Part print with two shaded views. Sizes in mm from the minimum x, y, z corner. A direction names the side the tool comes from. Give positions to 0.01 mm unless a question says otherwise; leave off trailing zeros. Order: outer loops, then holes, each group sorted by start corner. A loop starts at its lowest first (then second) coordinate and runs counter-clockwise, first axis right, second up. Notation, with made-up numbers: (70, -15.5) -> (127, -15.5) arc R17 cw to (127, -2.5) -> close; hole circle Ø4 at (-17.75, 39.5). An arc over 180 degrees is marked (long way). Write item = value, one per line. Start each with the question number.
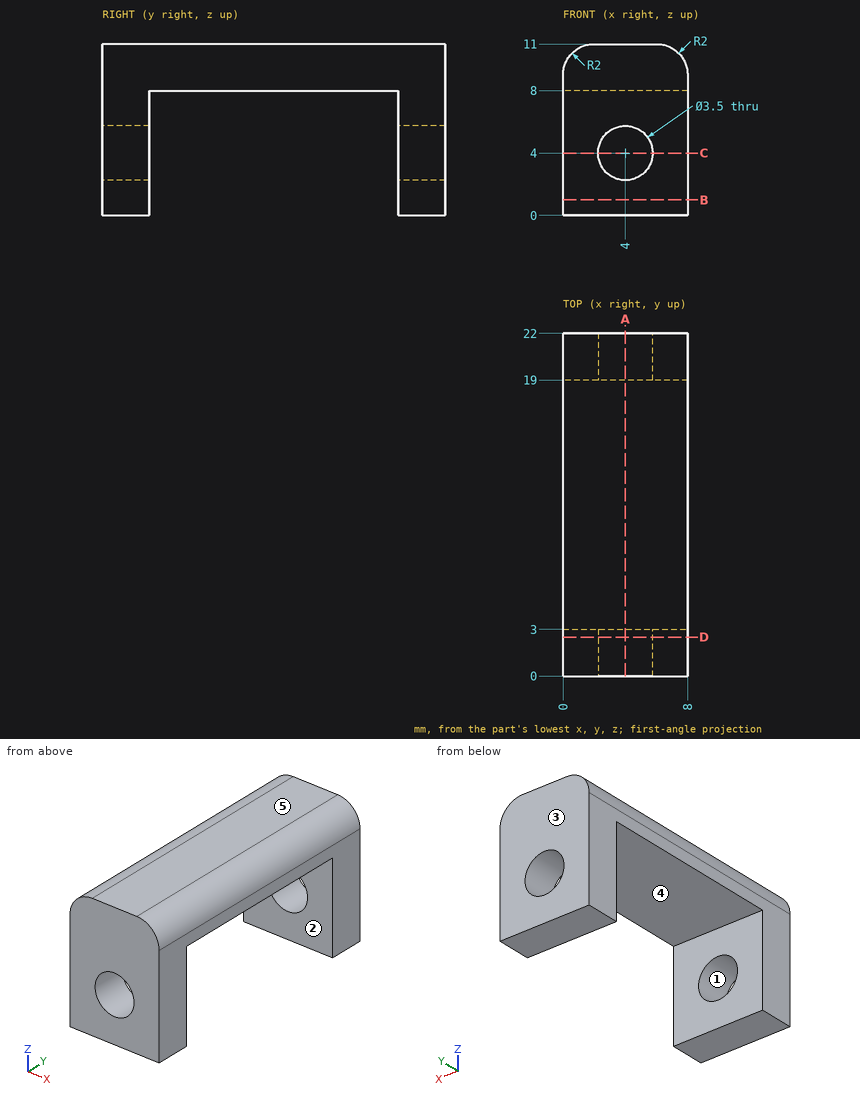
(1) Flat gauge pins, fed straight in: P1, Ø4, axis at x = 7, y = 15, coming from the +Z side; P2, Ø1, axis at x = 1, y = 9, coming from the -Z side. Where does each tip first touch, or does it go through?
(2) Cut at B-B, the plane z = 1. Give the cut face in (x, y).
(3) Cut at A-A, the plane x = 4. Give the cut face in (y, z).
(4) Cut at C-C, the plane z = 4. Give the cut face in (x, y), plus the area to 3 significant figures.
(5) 3-axis set-ups, long thin cutter, end or side, ignore diameter. For the marked faces 4 and 5: which of +Z, -Z, +X, -X, +Y, -Y reach the whole face in a straight line?
(6) Wall check: line 1 (Z direction, x = 4, y = 19.95); line 2 (Y direction, x = 1.75, z = 2.25); line 3 (X direction, y = 21.3, z = 4). Give the ranges that are in metal, low to high. Write a range as [from, to].
(7) Cut at D-D, the plane y = 2.5. Give the cut face in (x, z), plus the area to 3 significant figures.
(8) Mould opens along Y. For the marked faces 1, 2 and 3 say: released by +Y, released by -Y, zero draft, split by the parting line, or undercut.
Results:
q1.P1 = 11
q1.P2 = 8
q2.outline = (0, 0) -> (8, 0) -> (8, 3) -> (0, 3) -> close; (0, 19) -> (8, 19) -> (8, 22) -> (0, 22) -> close
q3.outline = (0, 0) -> (3, 0) -> (3, 2.25) -> (0, 2.25) -> close; (0, 5.75) -> (3, 5.75) -> (3, 8) -> (19, 8) -> (19, 5.75) -> (22, 5.75) -> (22, 11) -> (0, 11) -> close; (19, 0) -> (22, 0) -> (22, 2.25) -> (19, 2.25) -> close
q4.outline = (0, 0) -> (2.25, 0) -> (2.25, 3) -> (0, 3) -> close; (0, 19) -> (2.25, 19) -> (2.25, 22) -> (0, 22) -> close; (5.75, 0) -> (8, 0) -> (8, 3) -> (5.75, 3) -> close; (5.75, 19) -> (8, 19) -> (8, 22) -> (5.75, 22) -> close
q4.area = 27.0 mm2
q5.face_4 = -Z, +X, -X
q5.face_5 = +Z, +X, -X, +Y, -Y
q6.line_1 = [0, 2.25], [5.75, 11]
q6.line_2 = [0, 3], [19, 22]
q6.line_3 = [0, 2.25], [5.75, 8]
q7.outline = (0, 0) -> (8, 0) -> (8, 9) arc R2 ccw to (6, 11) -> (2, 11) arc R2 ccw to (0, 9) -> close; hole circle Ø3.5 at (4, 4)
q7.area = 76.7 mm2
q8.face_1 = zero draft
q8.face_2 = undercut
q8.face_3 = released by +Y
